Part model, mm, in its own coordinate system. A direction names the side the tool comes from. Coordinates: 2 decimals unless noted, no trailing zeros. Order: outer loops, then holes, each group sorted by start corner. A loop starts at its lowest first (then second) coordinate and runs counter-clockwise, first axis right, second up. Notation, with made-up numbers: (15.5, 11) - (32.5, 11) arc R29 ccw to (32.5, 39) - close; hole circle Ø10 at (-33, -1). An arc over 180 degrees is marked (long way). Use a Markdown table: item, result. Add a question column.
1) Saw through at D-D on x = 5. List the corners of the cut face in (y, z), then the cut area to 3 significant figures.
2) Saw through at C-C on z = 66. List the corners of the cut face in (x, y), then the cut area to 3 significant figures.
3) Saw through at A-A on x = 0. List the corners of the cut face in (y, z) (3 decimals), then the cut area to 3 significant figures.
4) Wall check: L1, parallel to Y at x = 0, z = 70; L2, parallel to Z at x = -7, y = -6.25; L3, parallel to Y at x = 0.5, z = 62. Give the ranges that are in metal, low to high. Write a range as [from, to].
5) Drop flat-ended pins along their axis: P1, Ø2, axis at x = -9.5, z = 24.5, coming from the +Y side; P2, Ø3, axis at y = -3, z = 25, coming from the +X side; P3, Ø4, axis at x = 7.5, z = 65, coming from the +Y side (3 decimals). Give the stop position or say it passes through.
6) Tool access for faces 1 (the face through (2, -2, 67.4)), 2 (the face through (0, 0, 0)), 3 (the face through (-8.922, -8.181, 7.888)): list every direction of +Z, -Z, +X, -X, +Y, -Y with a clear straight run to the whole face (end or side of a thin tool).
Autodesk Inventor part; units mm, degrees
ref_plane "YZ Plane" through (0, 0, 0) normal (1, 0, 0) x (0, 1, 0)
ref_plane "XZ Plane" through (0, 0, 0) normal (0, 1, 0) x (-1, 0, 0)
ref_plane "XY Plane" through (0, 0, 0) normal (0, 0, 1) x (1, 0, 0)
sketch "Sketch1" plane through (0, 0, 0) normal (0, 0, 1) x (1, 0, 0)
  circle A0 centre (0, 0) radius 12.105
  dimension "d0" = 24.21
extrude "Extrusion1" add sketch "Sketch1" along normal blind 16
sketch "Sketch2" plane through (0, 0, 16) normal (0, 0, 1) x (1, 0, 0)
  circle A0 centre (0, 0) radius 12.15
  dimension "d14" = 24.3
extrude "Extrusion2" add sketch "Sketch2" along normal blind 30
sketch "Sketch3" plane through (0, 0, 46) normal (0, 0, 1) x (1, 0, 0)
  circle A0 centre (0, 0) radius 12.5
  dimension "d5" = 25
extrude "Extrusion3" add sketch "Sketch3" along normal blind 19
sketch "Sketch4" plane through (0, 0, 65) normal (0, 0, 1) x (1, 0, 0)
  circle A0 centre (0, 0) radius 3.5
  dimension "d8" = 7
extrude "Extrusion4" add sketch "Sketch4" along normal blind 2.4
sketch "Sketch5" plane through (0, 0, 67.4) normal (0, 0, 1) x (1, 0, 0)
  circle A0 centre (0, 0) radius 2
  dimension "d11" = 4
extrude "Extrusion5" add sketch "Sketch5" along normal blind 11
properties part number "gearmotor" material "ABS Plastic"
Results are:
| question | item | result |
|---|---|---|
| 1 | outline | (-11.46, 46) - (-11.07, 46) - (-11.07, 16) - (-11.02, 16) - (-11.02, 0) - (11.02, 0) - (11.02, 16) - (11.07, 16) - (11.07, 46) - (11.46, 46) - (11.46, 65) - (-11.46, 65) - close |
| 1 | area | 1,450 mm2 |
| 2 | outline | circle Ø7 at (0, 0) |
| 2 | area | 38.5 mm2 |
| 3 | outline | (-12.5, 46) - (-12.15, 46) - (-12.15, 16) - (-12.105, 16) - (-12.105, 0) - (12.105, 0) - (12.105, 16) - (12.15, 16) - (12.15, 46) - (12.5, 46) - (12.5, 65) - (3.5, 65) - (3.5, 67.4) - (2, 67.4) - (2, 78.4) - (-2, 78.4) - (-2, 67.4) - (-3.5, 67.4) - (-3.5, 65) - (-12.5, 65) - close |
| 3 | area | 1,650 mm2 |
| 4 | L1 | [-2, 2] |
| 4 | L2 | [0, 65] |
| 4 | L3 | [-12.49, 12.49] |
| 5 | P1 | y = 8.68 |
| 5 | P2 | x = 12.06 |
| 5 | P3 | y = 11.225 |
| 6 | face 1 | +Z |
| 6 | face 2 | -Z, +X, -X, +Y, -Y |
| 6 | face 3 | -Z |
